Study the drawing (mm; zero at the part's minimum x, y, z) and answer. A direction names the side the tool comes from. Coordinates: 2 decimals unless noted, no trailing zeros. Order: outer loops, then holes, each group sorted by start corner. A loop starts at its lowest first (then second) coordinate and runs counter-clockwise, first axis right, second up.
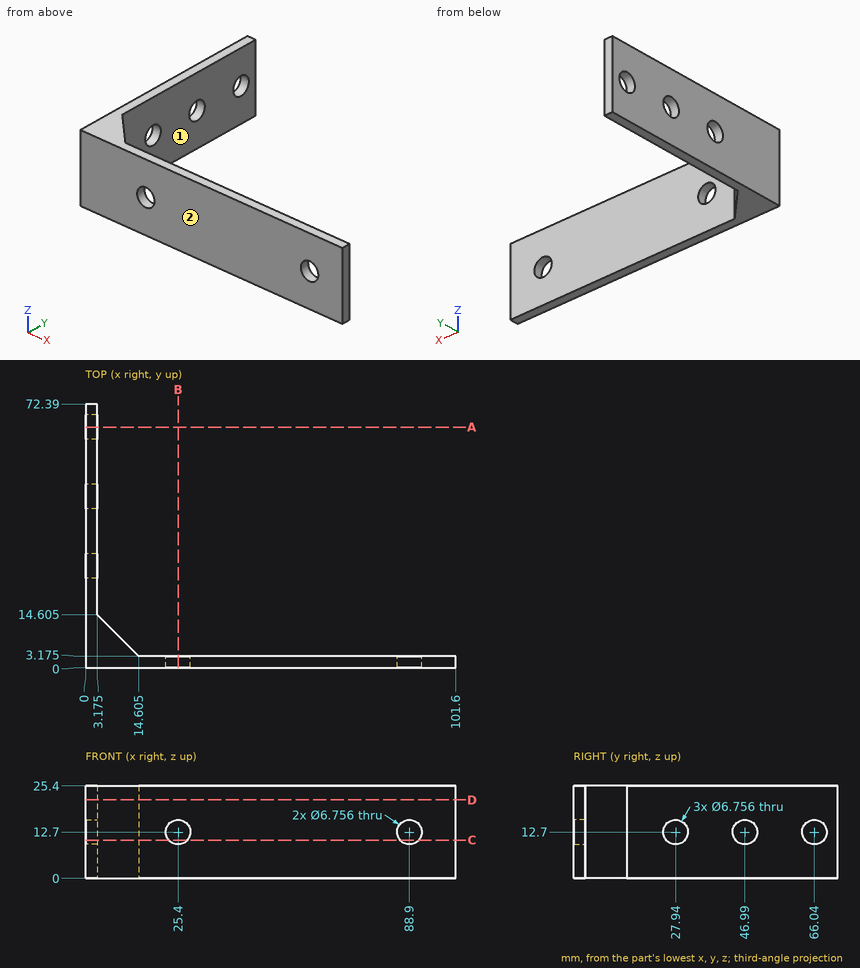
(1) For the marked faces 1 and 2, determine the directions among +Z, -Z, +X, -X, +Y, -Y from which every point of the face is accessible in a straight line to the end or side of a thin tool.
(2) Consider line 1 (Y direction, x = 0.7, z = 12.7); line 2 (X direction, y = 0.9, z = 12.7); line 3 (Z direction, x = 25, y = 2) (1 decimal). Determine where each line is inside the solid, lowest interval first.
(3) Each of these flat-tipped pins is pushed along its axis until it touches: pin 1 Ø11 at (x, z) = (25.4, 12.7) entering from +Y (3 decimals); pin 2 Ø1.5 at (y, z) = (38.5, 13) entering from +X (3 decimals); pin 3 Ø6 at (y, z) = (27.94, 12.7) entering from +X. Where does it stop, or does it pass through?
(4) Find section D-D (z = 21.5). Write down the section's boundary in (x, y) (1 decimal).
(5) Find section C-C (z = 10.5). Write down the section's boundary in (x, y) (1 decimal).
(6) Find section A-A (y = 66.04). Write down the section's boundary in (x, z) (1 decimal).
Findings below:
1. face 1: +Z, -Z, +X, +Y
1. face 2: +Z, -Z, +X, -X, -Y
2. line 1: y = 0 to 24.56, 31.32 to 43.61, 50.37 to 62.66, 69.42 to 72.39
2. line 2: x = 0 to 22.02, 28.78 to 85.52, 92.28 to 101.6
2. line 3: z = 0 to 9.3, 16.1 to 25.4
3. pin 1: stops at y = 3.175
3. pin 2: stops at x = 3.175
3. pin 3: passes through
4. outline: (0, 0) - (101.6, 0) - (101.6, 3.2) - (14.6, 3.2) - (3.2, 14.6) - (3.2, 72.4) - (0, 72.4) - close
5. outline: (0, 0) - (22.8, 0) - (22.8, 3.2) - (14.6, 3.2) - (3.2, 14.6) - (3.2, 25.4) - (0, 25.4) - close; (0, 30.5) - (3.2, 30.5) - (3.2, 44.4) - (0, 44.4) - close; (0, 49.6) - (3.2, 49.6) - (3.2, 63.5) - (0, 63.5) - close; (0, 68.6) - (3.2, 68.6) - (3.2, 72.4) - (0, 72.4) - close; (28, 0) - (86.3, 0) - (86.3, 3.2) - (28, 3.2) - close; (91.5, 0) - (101.6, 0) - (101.6, 3.2) - (91.5, 3.2) - close
6. outline: (0, 0) - (3.2, 0) - (3.2, 9.3) - (0, 9.3) - close; (0, 16.1) - (3.2, 16.1) - (3.2, 25.4) - (0, 25.4) - close
